The model under review builds one solid part; all positions refer to its coordinate system, in mm. Round coordinates to 2 decimals unless told otherwise and drop trailing zeros. Order: outer loops, then holes, each group sorted by start corner. A loop starts at its lowest first (then second) coordinate and runs counter-clockwise, first axis right, second up.
1) To check wall thickness, follow L1, parallel to Y at x = 97.5, z = 1.2; L2, parallel to X at y = -145, z = 2.4; L3, parallel to X at y = -230, z = 1.8. State the ranges of each line that lie inside material, in increasing order.
2) Consider section C-C (y = -93). Give the boundary of the cut face in (x, z).
3) Consider section A-A (y = -52.5). Give the boundary of the cut face in (x, z), then the cut area to 3 significant figures.
4) Consider section B-B (z = 0.75). Give the number of separate pieces and of enclosed holes in the cut face, then the cut area to 3 significant figures.
5) Clearance check with flat-ended pins moving along their axes: P1, Ø1.5, axis at y = -108.5, z = 2, coming from the +X side; P2, Ø3, axis at y = -198, z = 3, coming from the -X side; P3, Ø2.5, axis at x = -3.5, z = 2, coming from the -Y side. State where each tip first meets the part, or that it passes through.
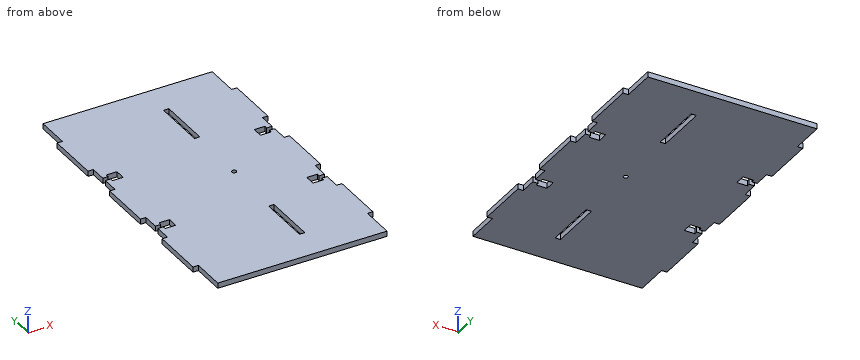
from build123d import *

# Parameters (mm, degrees)
ESQUISSE1_R        = 2.1
ESQUISSE1_W        = 5
ESQUISSE1_H        = 50
BOSS_EXTRU_1_DEPTH = 5


with BuildPart() as part:
    # Esquisse1 → Boss.-Extru.1 (new body)
    with BuildSketch(Plane.XY):
        Polygon((0, -3.53), (0, -35), (-5, -35), (-5, -85), (0, -85), (0, -100.4), (5, -100.4), (5, -97.5), (15, -97.5), (15, -107.5), (5, -107.5), (5, -104.6), (0, -104.6), (0, -120), (-5, -120), (-5, -170), (0, -170), (0, -185.4), (5, -185.4), (5, -182.5), (15, -182.5), (15, -192.5), (5, -192.5), (5, -189.6), (0, -189.6), (0, -205), (-5, -205), (-5, -255), (0, -255), (0, -286.47), (158.918484905, -286.47), (158.918484905, -255), (163.918484905, -255), (163.918484905, -205), (158.918484905, -205), (158.918484905, -189.6), (153.918484905, -189.6), (153.918484905, -192.5), (143.918484905, -192.5), (143.918484905, -182.5), (153.918484905, -182.5), (153.918484905, -185.4), (158.918484905, -185.4), (158.918484905, -170), (163.918484905, -170), (163.918484905, -120), (158.918484905, -120), (158.918484905, -104.6), (153.918484905, -104.6), (153.918484905, -107.5), (143.918484905, -107.5), (143.918484905, -97.5), (153.918484905, -97.5), (153.918484905, -100.4), (158.918484905, -100.4), (158.918484905, -85), (163.918484905, -85), (163.918484905, -35), (158.918484905, -35), (158.918484905, -3.53), align=None)
        with Locations((97.5, -145)):
            Circle(ESQUISSE1_R, mode=Mode.SUBTRACT)
        with Locations((97.5, -60)):
            Rectangle(ESQUISSE1_W, ESQUISSE1_H, mode=Mode.SUBTRACT)
        with Locations((97.5, -230)):
            Rectangle(ESQUISSE1_W, ESQUISSE1_H, mode=Mode.SUBTRACT)
    extrude(amount=BOSS_EXTRU_1_DEPTH)


solid = part.part
Answer below:
1. L1: y = -286.47 to -255, -205 to -147.1, -142.9 to -85, -35 to -3.53
1. L2: x = -5 to 95.4, 99.6 to 163.92
1. L3: x = -5 to 95, 100 to 163.92
2. outline: (0, 0) - (158.92, 0) - (158.92, 5) - (0, 5) - close
3. outline: (-5, 0) - (95, 0) - (95, 5) - (-5, 5) - close; (100, 0) - (163.92, 0) - (163.92, 5) - (100, 5) - close
3. area: 820 mm2
4. separate pieces: 1
4. enclosed holes: 3
4. area: 45,500 mm2
5. P1: stops at x = 158.92
5. P2: stops at x = 0
5. P3: stops at y = -255
